Geometry: see drawing. Coordinates: mm, zero at the bounding-box minimum. A direction names the side the tool comes from. Coordinates: 2 decimals unless noted, no trailing zeros. Write each loop counter-clockwise with the first axis right and the second up, starting at its lowest first coordinate (ties: lowest second). Pieces come first, ordered by that corner, then holes.
1) Pin query (flat end, axial travel): pin 1 Ø1.8 at (x, z) = (10, 10) entering from -Y; pin 2 Ø1.5 at (x, y) = (16.5, 1.5) entering from +Z; pin 3 Ø3.5 at (x, z) = (10, 16.75) entering from +Y; pin 4 Ø2 at (y, z) = (1.5, 15.5) entering from +X. Return the tip coordinate at first contact, or that it passes through.
2) Draft query along Z for the marked faces 3, 4 and 5. Return one class per face: pulls with the +Z half, pulls with the -Z half, needs draft (parallel to the pull), parting line crosses it, or undercut.
3) Section query C-C (y = 2.8). Output: boundary loops of the cut face in (x, z).
4) Section query A-A (x = 10). Output: boundary loops of the cut face in (y, z).
5) Set-up query: the marked faces 1 and 2. Return all of +Z, -Z, +X, -X, +Y, -Y with unobstructed straight access to the full face (end or side cutting, diameter ignored); none if empty.
6) Section query B-B (z = 10). Output: boundary loops of the cut face in (x, y).
7) Line query: L1, parallel to Z at x = 9.5, y = 0.55; L2, parallel to Z at x = 10, y = 2.55. Output: solid intervals per line, ascending.
8) Section query D-D (z = 3.25). Output: boundary loops of the cut face in (x, y), then the cut area to 3 significant figures.
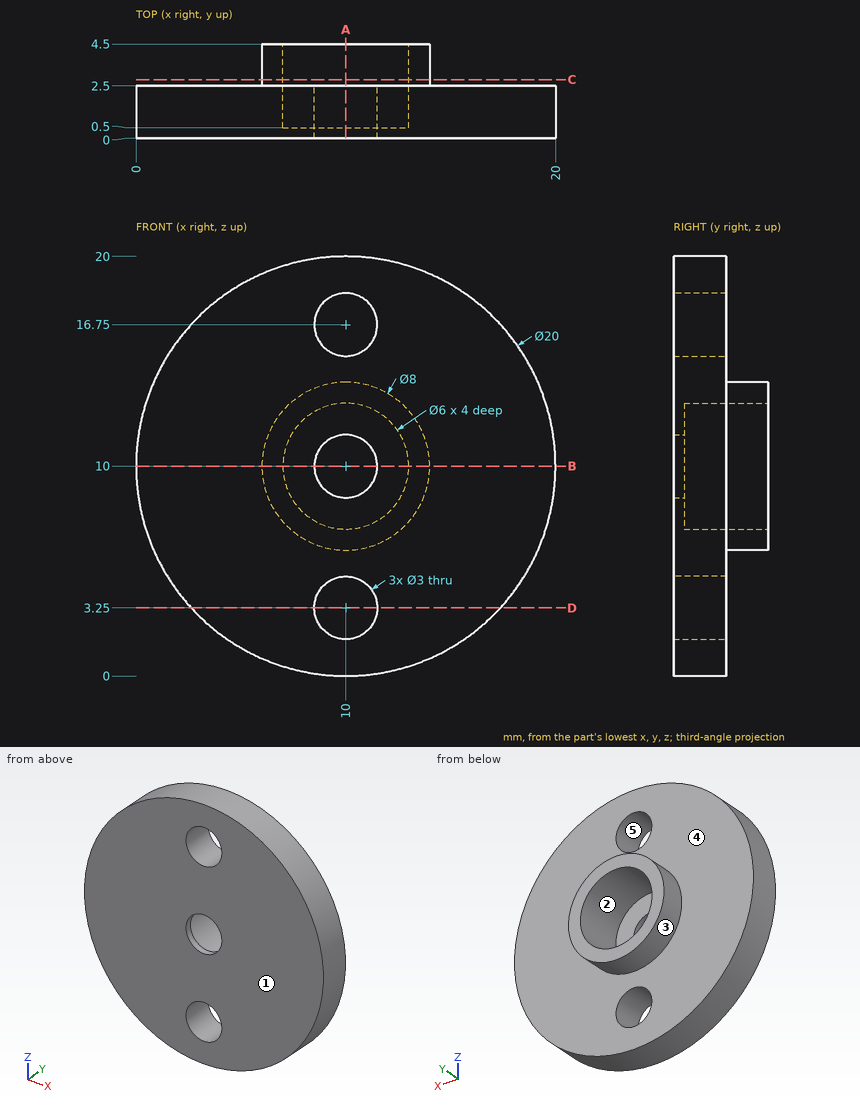
Answer:
1. pin 1: passes through
1. pin 2: stops at z = 18.18
1. pin 3: stops at y = 2.5
1. pin 4: stops at x = 18.93
2. face 3: parting line crosses it
2. face 4: needs draft
2. face 5: undercut
3. outline: circle Ø8 at (10, 10); hole circle Ø6 at (10, 10)
4. outline: (0, 0) - (2.5, 0) - (2.5, 1.75) - (0, 1.75) - close; (0, 4.75) - (2.5, 4.75) - (2.5, 6) - (4.5, 6) - (4.5, 7) - (0.5, 7) - (0.5, 8.5) - (0, 8.5) - close; (0, 11.5) - (0.5, 11.5) - (0.5, 13) - (4.5, 13) - (4.5, 14) - (2.5, 14) - (2.5, 15.25) - (0, 15.25) - close; (0, 18.25) - (2.5, 18.25) - (2.5, 20) - (0, 20) - close
5. face 1: +Z, -Z, +X, -X, -Y
5. face 2: +Y
6. outline: (0, 0) - (8.5, 0) - (8.5, 0.5) - (7, 0.5) - (7, 4.5) - (6, 4.5) - (6, 2.5) - (0, 2.5) - close; (11.5, 0) - (20, 0) - (20, 2.5) - (14, 2.5) - (14, 4.5) - (13, 4.5) - (13, 0.5) - (11.5, 0.5) - close
7. L1: z = 0.01 to 1.84, 4.66 to 7.04, 12.96 to 15.34, 18.16 to 19.99
7. L2: z = 6 to 7, 13 to 14
8. outline: (2.62, 0) - (8.5, 0) - (8.5, 2.5) - (2.62, 2.5) - close; (11.5, 0) - (17.38, 0) - (17.38, 2.5) - (11.5, 2.5) - close
8. area: 29.4 mm2
